Check sheet for the drawn part. Datum: minimum x, y, z corner. Units: mm. Coordinates: 2 decimals unless noted, no trailing zeros. Order: outer loops, then holes, each group sorted by start corner. A loop starts at its lowest first (then second) coordinate and runs counter-clockwise, first axis right, second up. Notation, with made-up numbers: M -3.75,-13 L 53.25,-13 A18 ccw 53.25,10 Z; hole C 14,-4.75 d2. An arc over 180 degrees is marked long. Return JSON: item names as keys, results as strings. Group by question number.
Q1. Section check B-B, the plane x = 99.5. Enter the section's corners in (y, z), then the cut area to 3 significant figures.
Q2. Section check A-A, the plane z = 6. Enter the section's corners in (x, y), then the cut area to 3 significant figures.
Q3. Thickness scan on probe 1 along Y at (x, z) = (254, 6.5); probe 2 along X at (y, z) = (533.4, 5); probe 3 along Y at (x, z) = (136, 13.75). Record the ranges inside material, lowest first.
Q4. Section check C-C, the plane y = 565. Enter the section's corners in (x, z).
Q5. Go/stop test with flat-tipped pins: pin 1 Ø1 at (y, z) = (378, 2) entering from +X; pin 2 Ø15 at (x, y) = (254, 533.4) entering from -Z; pin 3 Ø2 at (x, z) = (75, 4.5) entering from +Y; pin 4 Ø2 at (x, z) = (354.5, 2.5) entering from +Y. Record where each tip stops, or that it passes through.
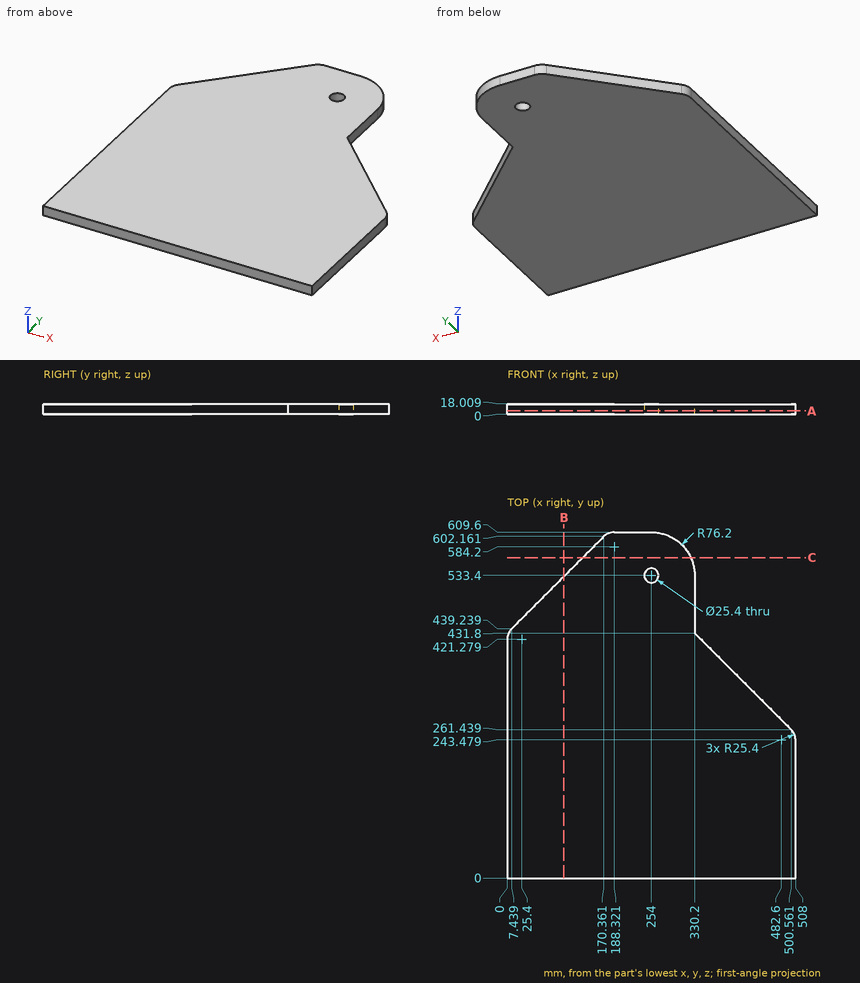
Numbers:
{
 "1": {"outline": "M 0,0 L 531.3,0 L 531.3,18.01 L 0,18.01 Z", "area": "9,570 mm2"},
 "2": {"outline": "M 0,0 L 508,0 L 508,243.48 A25.4 ccw 500.56,261.44 L 330.2,431.8 L 330.2,533.4 A76.2 ccw 254,609.6 L 188.32,609.6 A25.4 ccw 170.36,602.16 L 7.44,439.24 A25.4 ccw 0,421.28 Z; hole C 254,533.4 d25.4", "area": "245,000 mm2"},
 "3": {"probe 1": "y = 0 to 520.7, 546.1 to 609.6", "probe 2": "x = 101.6 to 241.3, 266.7 to 330.2", "probe 3": "y = 0 to 567.8"},
 "4": {"outline": "M 133.2,0 L 323.34,0 L 323.34,18.01 L 133.2,18.01 Z"},
 "5": {"pin 1": "stops at x = 384.5", "pin 2": "passes through", "pin 3": "stops at y = 507.8", "pin 4": "stops at y = 408.5"}
}
